```python
from build123d import *
from build123d import SkipClean  # not in build123d's __all__

# Parameters (mm, degrees)
F0_W      = 127
F0_H      = 127
F1_DEPTH  = 127
F2_R      = 38.1
F3_DEPTH  = 76.2
F4_R      = 38.1
F6_DEPTH  = 76.2
F7_R      = 38.1
F9_DEPTH  = 76.2
F10_R     = 38.1
F11_DEPTH = 76.2
F12_R     = 38.1
F13_DEPTH = 76.2
F14_R     = 38.1
F15_DEPTH = 76.2


with BuildPart() as f1:
    # F0 (on Front) → F1 (new body)
    with BuildSketch(Plane.XZ):
        with Locations((63.5, 63.5)):
            Rectangle(F0_W, F0_H)
    extrude(amount=F1_DEPTH)

    # F2 (on face) → F3 (cut)
    with BuildSketch(Plane.XZ.offset(127)):
        with Locations((63.5, 63.5)):
            Circle(F2_R)
    extrude(amount=-F3_DEPTH, mode=Mode.SUBTRACT)

    # F4 (on face) → F6 (cut)
    with BuildSketch(Plane(origin=(0, 0, 0), x_dir=(0, -1, 0), z_dir=(-1, 0, 0))):
        with Locations((63.5, 63.5)):
            Circle(F4_R)
    extrude(amount=-F6_DEPTH, mode=Mode.SUBTRACT)

    # F7 (on face) → F9 (cut)
    with BuildSketch(Plane.YZ.offset(127)):
        with Locations((-63.5, 63.5)):
            Circle(F7_R)
    with SkipClean():  # cleaning this boolean's faces spoils the solid; the shape is the same uncleaned
        extrude(amount=-F9_DEPTH, mode=Mode.SUBTRACT)

    # F10 (on face) → F11 (cut)
    with BuildSketch(Plane(origin=(0, 0, 0), x_dir=(-1, 0, 0), z_dir=(0, 1, 0))):
        with Locations((-63.5, 63.5)):
            Circle(F10_R)
    extrude(amount=-F11_DEPTH, mode=Mode.SUBTRACT)

    # F12 (on face) → F13 (cut)
    with BuildSketch(Plane.XY.offset(127)):
        with Locations((62.3162926857, -62.3162926857)):
            Circle(F12_R)
    extrude(amount=-F13_DEPTH, mode=Mode.SUBTRACT)

    # F14 (on face) → F15 (cut)
    with BuildSketch(Plane(origin=(0, 0, 0), x_dir=(1, 0, 0), z_dir=(0, 0, -1))):
        with Locations((63.5, 63.5)):
            Circle(F14_R)
    extrude(amount=-F15_DEPTH, mode=Mode.SUBTRACT)


solid = f1.part
```
Could you check a few things on this model? Use its own coordinates, in mm. A direction names the side the tool comes from. Coordinates: 2 decimals unless noted, no trailing zeros. Write each loop counter-clockwise with the first axis right and the second up, starting at its lowest first coordinate (ties: lowest second). Pieces come first, ordered by that corner, then holes. Notation, with made-up numbers: (-7, 65.25) -> (7, 65.25) arc R23 cw to (7, 94.25) -> close; hole circle Ø6 at (89.25, 69). An arc over 180 degrees is marked (long way). Return JSON: item names as keys, results as strings.
(1) Imagine slicing it at C-C, the plane z = 23.5. Please give me the cut outline in (x, y), then the cut area to 3 significant figures.
Numbers:
{"outline": "(0, -127) -> (127, -127) -> (127, 0) -> (0, 0) -> close; hole circle Ø76.2 at (63.5, -63.5)", "area": "11,600 mm2"}
(2) I need wall thicknesses on L1, parallel to Z at x = 15, y = -63; L2, parallel to Y at x = 105, z = 63. Which ranges of each line are inside material? Lowest first, please.
Numbers:
{"L1": "z = 0 to 25.4, 101.6 to 127", "L2": "y = -127 to -101.6, -25.4 to 0"}
(3) Imagine slicing it at B-B, the plane y = -68.5. Please give me the cut outline in (x, z), then the cut area to 3 significant figures.
Numbers:
{"outline": "(0, 0) -> (25.73, 0) -> (25.73, 25.73) -> (0, 25.73) -> close; (0, 101.27) -> (24.72, 101.27) -> (24.72, 127) -> (0, 127) -> close; (99.91, 101.27) -> (127, 101.27) -> (127, 127) -> (99.91, 127) -> close; (101.27, 0) -> (127, 0) -> (127, 25.73) -> (101.27, 25.73) -> close", "area": "2,660 mm2"}
(4) Imagine slicing it at D-D, the plane x = 14. Please give me the cut outline in (y, z).
Numbers:
{"outline": "(-127, 0) -> (0, 0) -> (0, 127) -> (-127, 127) -> close; hole circle Ø76.2 at (-63.5, 63.5)"}
(5) I'm going to push flat-ended pins straight in: pin 1 (1.5 mm diameter, centred on y = -75, z = 104, fed in from -X); pin 2 (12 mm diameter, centred on x = 33.5, y = -60.5, fed in from -Z). Where does each tip first touch, or does it pass through?
Numbers:
{"pin 1": "stops at x = 0", "pin 2": "passes through"}
(6) Which directions (+Z, -Z, +X, -X, +Y, -Y) give clear straight access to the entire face, cutting with the end or side of a thin tool? Please do faces 1 (the cylindrical face through (35.42, -89.25, 13.96)), 2 (the cylindrical face through (13.97, -35.42, 89.25)).
Numbers:
{"face 1": "-Z", "face 2": "+X, -X"}
(7) We'd pull the mould along Y, two halves only. Please class faces 3 (the cylindrical face through (34.235, -36.567, 112.566)), 4 (the flat face through (34, -127, 36)), 5 (the flat face through (34, -91, 0)), 6 (the flat face through (34, 0, 36)): +Y half, -Y half, draft (parallel to the pull), parting line (faces both ways), or undercut.
Numbers:
{"face 3": "undercut", "face 4": "-Y half", "face 5": "draft", "face 6": "+Y half"}
(8) Imagine slicing it at A-A, the plane z = 63.5. Please give me the cut outline in (x, y).
Numbers:
{"outline": "(0, -127) -> (25.4, -127) -> (25.4, -101.6) -> (0, -101.6) -> close; (0, -25.4) -> (25.4, -25.4) -> (25.4, 0) -> (0, 0) -> close; (101.6, -127) -> (127, -127) -> (127, -101.6) -> (101.6, -101.6) -> close; (101.6, -25.4) -> (127, -25.4) -> (127, 0) -> (101.6, 0) -> close"}
